Part model, mm, in its own coordinate system. Face numbers are marked on the shaded views. Round coordinates to 2 decimals unless told otherwise and drop trailing zeros. Write each loop counter-clockwise with the first axis right and the second up, starting at its lowest first coordinate (ties: lowest second). Pieces come first, ordered by that corner, then holes.
1) Drill centre lines: L1, parallel to Z at x = 22.5, y = 11; L2, parallel to Y at x = 103, z = 100.5. Where is each one in solid material? Low to high.
2) Saw through at B-B on x = 99. Write the cut outline in (y, z).
3) Flat gauge pins, fed straight in: pin 1 (1.6 mm diameter, centred on x = 53.5, y = 11, fed in from -Z); pin 2 (1.6 mm diameter, centred on y = 11, z = -1, fed in from +X); pin 3 (2 mm diameter, centred on x = 34, y = 11.5, fed in from +Z). Where does each tip first touch, or does it go through?
4) Saw through at A-A on z = 13. Write the cut outline in (x, y), and give its area (3 significant figures).
5) Pull direction Z, two halves, no side cores. Call the marked faces 1 and 2: +Z half, -Z half, draft (parallel to the pull), parting line (faces both ways), or undercut.
Autodesk Fusion 360 part; units mm, degrees
sketch "Sketch1" plane through (0, 0, 0) normal (0, 1, 0) x (1, 0, 0)
  line L0 (-50, 50) -> (130, 50)
  line L1 (130, 50) -> (130, -130)
  line L2 (130, -130) -> (-50, -130)
  line L3 (-50, -130) -> (-50, 50)
  dimension "d1" = 180
  dimension "d2" = 180
extrude "Extrude1" add sketch "Sketch1" along normal blind 10
sketch "Sketch2" plane through (0, 10, 0) normal (0, 1, 0) x (-1, 0, 0)
  line L0 (50, 130) -> (-130, 130)
  line L1 (-130, 130) -> (-130, -50)
  line L2 (-130, -50) -> (50, -50)
  line L3 (50, -50) -> (50, 130)
  line L4 (46, 126) -> (-126, 126)
  line L5 (-126, 126) -> (-126, -46)
  line L6 (-126, -46) -> (46, -46)
  line L7 (46, -46) -> (46, 126)
  dimension "d5" = 172
  dimension "d6" = 172
extrude "Extrude2" add sketch "Sketch2" along normal blind 2 contours L4 L5 L6 L7
sketch "Sketch3" plane through (0, 12, 0) normal (0, 1, 0) x (-1, 0, 0)
  line L0 (46, -46) -> (46, 126)
  line L1 (46, 126) -> (-126, 126)
  line L2 (-126, 126) -> (-126, -46)
  line L3 (-126, -46) -> (46, -46)
  line L4 (44, 124) -> (-124, 124)
  line L5 (-124, 124) -> (-124, -44)
  line L6 (-124, -44) -> (44, -44)
  line L7 (44, -44) -> (44, 124)
extrude "Extrude3" cut sketch "Sketch3" against normal blind 2 contours L4 L5 L6 L7
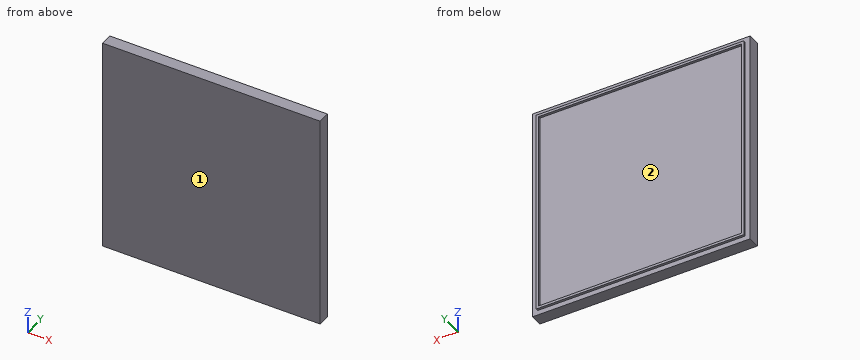
Completed:
1. L1: z = -46 to -44, 124 to 126
1. L2: y = 0 to 10
2. outline: (0, -50) - (10, -50) - (10, -46) - (12, -46) - (12, -44) - (10, -44) - (10, 124) - (12, 124) - (12, 126) - (10, 126) - (10, 130) - (0, 130) - close
3. pin 1: stops at z = -46
3. pin 2: stops at x = 126
3. pin 3: stops at z = 126
4. outline: (-50, 0) - (130, 0) - (130, 10) - (126, 10) - (126, 12) - (124, 12) - (124, 10) - (-44, 10) - (-44, 12) - (-46, 12) - (-46, 10) - (-50, 10) - close
4. area: 1,810 mm2
5. face 1: draft
5. face 2: undercut
